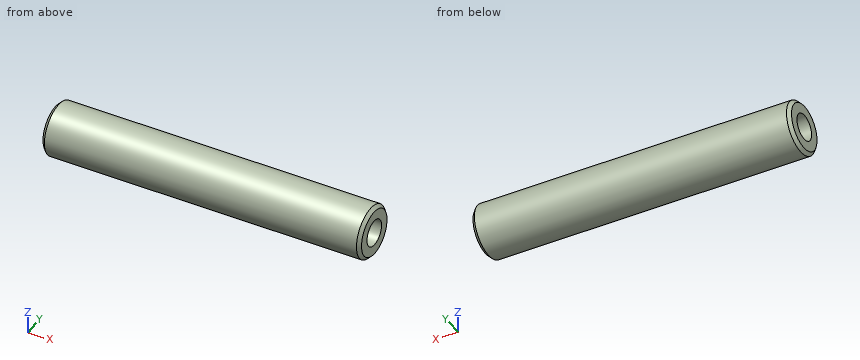
```python
from build123d import *

# Parameters (mm, degrees)
SKETCH_1_W                     = 49.2
SKETCH_1_H                     = 4
M4X0_7_1_D                     = 3.3
M4X0_7_1_DEPTH                 = 11.5
M4X0_7_1_CBORE_D               = 4
M4X0_7_1_CBORE_DEPTH           = 8
M4X0_7_1_TIP                   = 0.991420021
M4X0_7_1_ON_FACE_2_D           = 3.3
M4X0_7_1_ON_FACE_2_DEPTH       = 11.5
M4X0_7_1_ON_FACE_2_CBORE_D     = 4
M4X0_7_1_ON_FACE_2_CBORE_DEPTH = 8
M4X0_7_1_ON_FACE_2_TIP         = 0.991420021
CHAMFER_1_SIZE                 = 0.5


with BuildPart() as part:
    # ｽｹｯﾁ1 → 回転1 (revolve)
    with BuildSketch(Plane.XY, mode=Mode.PRIVATE) as revolve_1_sk:
        with Locations((0, 2)):
            Rectangle(SKETCH_1_W, SKETCH_1_H)
    revolve(revolve_1_sk.sketch.rotate(Axis((0, 0, 0), (1, 0, 0)), 90), axis=Axis((0, 0, 0), (1, 0, 0)))

    # M4x0.7 ねじ穴1
    with Locations(Plane(origin=(24.6, 0, 0), x_dir=(0, 0, 1), z_dir=(1, 0, 0))):
        with Locations((0, 0)):
            CounterBoreHole(M4X0_7_1_D / 2, M4X0_7_1_CBORE_D / 2, M4X0_7_1_CBORE_DEPTH, depth=M4X0_7_1_DEPTH)
            with Locations((0, 0, -(M4X0_7_1_DEPTH + M4X0_7_1_TIP / 2))):  # 118° drill point
                Cone(0, M4X0_7_1_D / 2, M4X0_7_1_TIP, mode=Mode.SUBTRACT)

    # M4x0.7 ねじ穴1 on face 2
    with Locations(Plane(origin=(-24.6, 0, 0), x_dir=(0, 0, -1), z_dir=(-1, 0, 0))):
        with Locations((0, 0)):
            CounterBoreHole(M4X0_7_1_ON_FACE_2_D / 2, M4X0_7_1_ON_FACE_2_CBORE_D / 2, M4X0_7_1_ON_FACE_2_CBORE_DEPTH, depth=M4X0_7_1_ON_FACE_2_DEPTH)
            with Locations((0, 0, -(M4X0_7_1_ON_FACE_2_DEPTH + M4X0_7_1_ON_FACE_2_TIP / 2))):  # 118° drill point
                Cone(0, M4X0_7_1_ON_FACE_2_D / 2, M4X0_7_1_ON_FACE_2_TIP, mode=Mode.SUBTRACT)

    # 面取り1
    chamfer_1_edges = [part.edges().sort_by_distance(p)[0] for p in [
        (24.6, 0, -4),
        (-24.6, 0, -4),
    ]]
    chamfer(chamfer_1_edges, length=CHAMFER_1_SIZE)


solid = part.part
```
Design review of the part built by this model. Coordinates are the model's own, in mm. Coordinates: 2 decimals unless noted, no trailing zeros. Order: outer loops, then holes, each group sorted by start corner. A loop starts at its lowest first (then second) coordinate and runs counter-clockwise, first axis right, second up. Notation, with made-up numbers: (78, -21) - (103, -21) arc R27 ccw to (103, 11) - close; hole circle Ø8 at (-39, 23.5). An arc over 180 degrees is marked (long way). Answer in a Markdown table with one row per item.
(1) Wall thickness on line 1 along Y through (x, z) = (-14.95, 0); line 2 along Y through (x, z) = (21.5, 0); line 3 along Z through (x, y) = (17, -2.75): over which ranges is each line inside the solid? List them lowest first. Write a range as from..to.
Checked values:
| item | result |
|---|---|
| line 1 | -4..-1.65, 1.65..4 |
| line 2 | -4..-2, 2..4 |
| line 3 | -2.9..2.9 |
(2) Clearance check with flat-ended pins moving along their axes: pin 1 (2 mm diameter, centred on y = 0, z = -0.5, fed in from -X); pin 2 (1 mm diameter, centred on x = 2, y = -2.5, fed in from -Z); pin 3 (1 mm diameter, centred on x = 2, z = -3, fed in from +Y). State where each tip first meets the part, or that it passes through.
Checked values:
| item | result |
|---|---|
| pin 1 | x = -13.01 |
| pin 2 | z = -3.46 |
| pin 3 | y = 3.12 |
(3) Consider section A-A on x = -15.5. State the section outline as (y, z) points.
Checked values:
| item | result |
|---|---|
| outline | circle Ø8 at (0, 0); hole circle Ø3.3 at (0, 0) |
(4) Consider section B-B on x = 4. State the section outline as (y, z) points.
Checked values:
| item | result |
|---|---|
| outline | circle Ø8 at (0, 0) |
